from build123d import *
from OCP.BRepFilletAPI import BRepFilletAPI_MakeChamfer

# Parameters (mm, degrees)
BOSS_EXTRUDE1_DEPTH     = 23.2
BOSS_EXTRUDE2_START     = 23.2
BOSS_EXTRUDE2_DEPTH     = 75
CUT_EXTRUDE1_DEPTH      = 108.706127959
CUT_EXTRUDE1_DEPTH_BACK = 108.706127959
SKETCH2_W               = 2
SKETCH2_H               = 5
CUT_EXTRUDE2_DEPTH      = 108.706127959
CUT_EXTRUDE2_DEPTH_BACK = 108.706127959
CUT_EXTRUDE3_DEPTH      = 108.706127959
CUT_EXTRUDE3_DEPTH_BACK = 108.706127959
BOSS_EXTRUDE3_DEPTH     = 3.2
SKETCH5_W               = 84.2
SKETCH5_H               = 3.2
BOSS_EXTRUDE4_DEPTH     = 120
BOSS_EXTRUDE5_DEPTH     = 120
CUT_EXTRUDE4_DEPTH      = 136.132897549
CUT_EXTRUDE4_DEPTH_BACK = 136.132897549
CHAMFER1_SIZE           = 3.6
CHAMFER1_SIZE2          = 1.2
CHAMFER2_SIZE           = 1.2
FILLET1_R               = 0.8


with BuildPart() as part:
    # Sketch1 → Boss-Extrude1 (new body)
    with BuildSketch(Plane(origin=(0, 0, 0), x_dir=(1, 0, 0), z_dir=(0, 1, 0))):
        Polygon((-22.25475327, 13.6), (22.25475327, 13.6), (42.1, 10.359959718), (42.1, -10.359959718), (22.25475327, -13.6), (-22.25475327, -13.6), (-42.1, -10.359959718), (-42.1, 10.359959718), align=None)
    extrude(amount=BOSS_EXTRUDE1_DEPTH)

    # Sketch1<3> → Boss-Extrude2 (add)
    with BuildSketch(Plane(origin=(0, 0, 0), x_dir=(1, 0, 0), z_dir=(0, 1, 0)).offset(BOSS_EXTRUDE2_START)):
        Polygon((40.5, -9), (28.25, -11), (28.25, -8.9), (11, -8.9), (11, -12), (-11, -12), (-11, -8.9), (-28.25, -8.9), (-28.25, -11), (-40.5, -9), (-40.5, 9), (-28.25, 11), (-28.25, 8.9), (-11, 8.9), (-11, 12), (11, 12), (11, 8.9), (28.25, 8.9), (28.25, 11), (40.5, 9), align=None)
        Polygon((-38.9, -7.640040282), (-29.85, -9.117591303), (-29.85, -7.3), (-9.4, -7.3), (-9.4, -10.4), (9.4, -10.4), (9.4, -7.3), (29.85, -7.3), (29.85, -9.117591303), (38.9, -7.640040282), (38.9, 7.640040282), (29.85, 9.117591303), (29.85, 7.3), (9.4, 7.3), (9.4, 10.4), (-9.4, 10.4), (-9.4, 7.3), (-29.85, 7.3), (-29.85, 9.117591303), (-38.9, 7.640040282), align=None, mode=Mode.SUBTRACT)
    extrude(amount=BOSS_EXTRUDE2_DEPTH)

    # Sketch2 → Cut-Extrude1 (cut, two sides: drawn at the far end of the back side and taken through both)
    with BuildSketch(Plane.XY.offset(-CUT_EXTRUDE1_DEPTH_BACK)):
        with Locations((-39.5, 44.7)):
            Rectangle(SKETCH2_W, SKETCH2_H)
        with Locations((39.5, 44.7)):
            Rectangle(SKETCH2_W, SKETCH2_H)
    extrude(amount=CUT_EXTRUDE1_DEPTH + CUT_EXTRUDE1_DEPTH_BACK, mode=Mode.SUBTRACT)

    # Sketch3 → Cut-Extrude2 (cut, two sides: drawn at the far end of the back side and taken through both)
    with BuildSketch(Plane.XY.offset(-CUT_EXTRUDE2_DEPTH_BACK)):
        Polygon((-28.25, 93.2), (-19.625, 23.2), (19.625, 23.2), (28.25, 93.2), (28.25, 98.2), (-28.25, 98.2), align=None)
    extrude(amount=CUT_EXTRUDE2_DEPTH + CUT_EXTRUDE2_DEPTH_BACK, mode=Mode.SUBTRACT)

    # Sketch1<4> → Cut-Extrude3 (cut, two sides: drawn at the far end of the back side and taken through both)
    with BuildSketch(Plane(origin=(0, 0, 0), x_dir=(1, 0, 0), z_dir=(0, 1, 0)).offset(-CUT_EXTRUDE3_DEPTH_BACK)):
        Polygon((-31.45, -5.7), (-7.8, -5.7), (-7.8, -8.8), (7.8, -8.8), (7.8, -5.7), (31.45, -5.7), (31.45, -7.235182606), (37.3, -6.280080565), (37.3, 6.280080565), (31.45, 7.235182606), (31.45, 5.7), (7.8, 5.7), (7.8, 8.8), (-7.8, 8.8), (-7.8, 5.7), (-31.45, 5.7), (-31.45, 7.235182606), (-37.3, 6.280080565), (-37.3, -6.280080565), (-31.45, -7.235182606), align=None)
    extrude(amount=CUT_EXTRUDE3_DEPTH + CUT_EXTRUDE3_DEPTH_BACK, mode=Mode.SUBTRACT)

    # Sketch4 → Boss-Extrude3 (add)
    with BuildSketch(Plane(origin=(0, 0, 0), x_dir=(1, 0, 0), z_dir=(0, 1, 0))):
        Polygon((42.1, 10.359959718), (22.25475327, 13.6), (-22.25475327, 13.6), (-42.1, 10.359959718), (-42.1, 42.5), (42.1, 42.5), align=None)
    extrude(amount=BOSS_EXTRUDE3_DEPTH)

    # Sketch5 → Boss-Extrude4 (add)
    with BuildSketch(Plane(origin=(0, 0, 0), x_dir=(1, 0, 0), z_dir=(0, 1, 0))):
        with Locations((0, 44.1)):
            Rectangle(SKETCH5_W, SKETCH5_H)
    extrude(amount=BOSS_EXTRUDE4_DEPTH)

    # Sketch6 → Boss-Extrude5 (add)
    with BuildSketch(Plane(origin=(0, 0, 0), x_dir=(1, 0, 0), z_dir=(0, 1, 0))):
        Polygon((-42.1, 42.5), (42.1, 42.5), (28.25, 40.9), (-28.25, 40.9), align=None)
    extrude(amount=BOSS_EXTRUDE5_DEPTH)

    # Sketch7 → Cut-Extrude4 (cut, two sides: drawn at the far end of the back side and taken through both)
    with BuildSketch(Plane(origin=(0, 0, 0), x_dir=(-1, 0, 0), z_dir=(0, 0, -1)).offset(-CUT_EXTRUDE4_DEPTH_BACK)):
        with BuildLine():
            Line((-12, 67.5), (-12, 52.5))
            ThreePointArc((-12, 52.5), (-15, 49.5), (-18, 52.5))
            Line((-18, 52.5), (-18, 67.5))
            ThreePointArc((-18, 67.5), (-15, 70.5), (-12, 67.5))
        make_face()
        with BuildLine():
            Line((12, 67.5), (12, 52.5))
            ThreePointArc((12, 52.5), (15, 49.5), (18, 52.5))
            Line((18, 52.5), (18, 67.5))
            ThreePointArc((18, 67.5), (15, 70.5), (12, 67.5))
        make_face()
    extrude(amount=CUT_EXTRUDE4_DEPTH + CUT_EXTRUDE4_DEPTH_BACK, mode=Mode.SUBTRACT)

    # Chamfer1: one chamfer whose edges measure the first distance from different faces: ONE call of the kernel's chamfer builder (chamfer() names one face for all edges)
    chamfer1_edges_1 = [part.edges().sort_by_distance(p)[0] for p in [
        (35.175, 120, -41.7),
    ]]
    chamfer1_side_1 = [part.faces().sort_by_distance(p)[0] for p in [
        (35.175, 61.6, -41.7),
    ]]
    chamfer1_edges_2 = [part.edges().sort_by_distance(p)[0] for p in [
        (0, 120, -40.9),
    ]]
    chamfer1_side_2 = [part.faces().sort_by_distance(p)[0] for p in [
        (0, 61.659484301, -40.9),
    ]]
    chamfer1_edges_3 = [part.edges().sort_by_distance(p)[0] for p in [
        (-35.175, 120, -41.7),
    ]]
    chamfer1_side_3 = [part.faces().sort_by_distance(p)[0] for p in [
        (-35.175, 61.6, -41.7),
    ]]
    chamfer1 = BRepFilletAPI_MakeChamfer(part.part.solid().wrapped)
    for e in chamfer1_edges_1:
        chamfer1.Add(CHAMFER1_SIZE, CHAMFER1_SIZE2, e.wrapped, chamfer1_side_1[0].wrapped)  # the first distance lies on this face
    for e in chamfer1_edges_2:
        chamfer1.Add(CHAMFER1_SIZE, CHAMFER1_SIZE2, e.wrapped, chamfer1_side_2[0].wrapped)  # the first distance lies on this face
    for e in chamfer1_edges_3:
        chamfer1.Add(CHAMFER1_SIZE, CHAMFER1_SIZE2, e.wrapped, chamfer1_side_3[0].wrapped)  # the first distance lies on this face
    add(Compound.cast(chamfer1.Shape()), mode=Mode.REPLACE)

    # Chamfer2
    chamfer2_edges = [part.edges().sort_by_distance(p)[0] for p in [
        (-42.1, 0, -17.670020141),
        (-7.8, 23.2, 7.25),
        (7.8, 23.2, 7.25),
        (7.8, 23.2, -7.25),
        (-7.8, 23.2, -7.25),
        (-7.8, 0, -7.25),
        (-7.8, 0, 7.25),
        (40.5, 98.2, 0),
        (28.25, 98.2, -9.15),
        (0, 0, -45.7),
        (-28.25, 98.2, 9.15),
        (28.25, 98.2, 9.15),
        (-28.25, 98.2, -9.15),
        (-40.5, 98.2, 0),
        (-32.177376635, 0, 11.979979859),
        (0, 0, 13.6),
        (32.177376635, 0, 11.979979859),
        (42.1, 0, -17.670020141),
    ]]
    chamfer(chamfer2_edges, length=CHAMFER2_SIZE)

    # Fillet1
    fillet1_edges = [part.edges().sort_by_distance(p)[0] for p in [
        (-42.1, 12.2, 10.359959718),
        (42.1, 12.2, 10.359959718),
        (42.1, 13.2, -10.359959718),
        (-42.1, 13.2, -10.359959718),
        (-42.1, 60.6, -45.7),
        (42.1, 60.6, -45.7),
    ]]
    fillet(fillet1_edges, radius=FILLET1_R)


solid = part.part
Design review of the part built by this model. Coordinates are the model's own, in mm. A direction names the side the tool comes from. Coordinates: 2 decimals unless noted, no trailing zeros. Loops run counter-clockwise (first coordinate to the right, second up) from the corner with the lowest first, then second, coordinate; pieces in that order, holes last. Notation, with made-up numbers: (88, 59) -> (112, 59) arc R19 cw to (112, 68) -> close; hole circle Ø9 at (57.5, 65). An arc over 180 degrees is marked (long way). Use a Markdown table: item, result. Add a question column.
Item 1: The part is to be moulded in two halves that separate along X. For faces 1 (the flat face through (1, 3.2, -26)), 2 (the flat face through (-28.25, 60, -10)), 3 (the flat face through (-31.708, 12.046, 12.057)), say which applies: +X half, -X half, draft (parallel to the pull), parting line (faces both ways), or undercut.
Item 2: Wall thickness on L1, parallel to Z at x = 3, y = 7; L2, parallel to Z at x = -24.5, y = 47; L3, parallel to X at y = 19, z = -8: over which ranges is each line inside the solid? List them lowest first. Write a range as from..to.
Item 3: Clearance check with flat-ended pins moving along their axes: P1, Ø10, axis at x = -1, z = -4.5, coming from the -Y side; P2, Ø12, axis at x = 23, y = 59, coming from the +Z side; P3, Ø0.8, axis at y = 45, z = 8, coming from the +X side; P4, Ø0.9, axis at y = 54.5, z = 8, coming from the -X side. State where each tip first meets the part, or that it passes through.
Item 4: Machinability: for faces 4 (the flat face through (31.708, 13.06, -12.057)), 5 (the flat face through (40.5, 33, 0)), 6 (the flat face through (20, 11, -5.7)), which of the approach directions +Z, -Z, +X, -X, +Y, -Y give a long, thin tool a straight path to every point of the face, cutting with its end or side? Answer none if there is none.
Item 5: We need section A-A, the plane z = 0.5. Write out the cut boundary in (x, y).
Item 6: We need section D-D, the plane y = 82. Count the separate pieces of the cut face and the enclosed holes in it, and give its area (3 significant figures).
Item 7: We need section C-C, the plane x = -2.5. Write out the cut boundary in (y, z), and give its area (3 significant figures).
Item 8: We need section B-B, the plane x = 15. Write out the cut boundary in (y, z).
Numbers:
| question | item | result |
|---|---|---|
| 1 | face 1 | draft |
| 1 | face 2 | undercut |
| 1 | face 3 | -X half |
| 2 | L1 | z = -45.7..-40.9, -13.6..-8.8, 8.8..13.6 |
| 2 | L2 | z = -45.7..-40.9, -8.9..-7.3, 7.3..8.9 |
| 2 | L3 | x = -42.1..-7.8, 7.8..42.1 |
| 3 | P1 | stops at y = 0 |
| 3 | P2 | stops at z = 11 |
| 3 | P3 | stops at x = 38.5 |
| 3 | P4 | stops at x = -40.5 |
| 4 | face 4 | +X, +Y |
| 4 | face 5 | +Z, +X, +Y |
| 4 | face 6 | +Y, -Y |
| 5 | outline | (-42.1, 1.2) -> (-40.9, 0) -> (-37.3, 0) -> (-37.3, 23.2) -> (-38.9, 23.2) -> (-38.9, 42.2) -> (-40.5, 42.2) -> (-40.5, 23.2) -> (-42.1, 23.2) -> close; (-40.5, 47.2) -> (-38.9, 47.2) -> (-38.9, 98.2) -> (-39.3, 98.2) -> (-40.5, 97) -> close; (37.3, 0) -> (40.9, 0) -> (42.1, 1.2) -> (42.1, 23.2) -> (40.5, 23.2) -> (40.5, 42.2) -> (38.9, 42.2) -> (38.9, 23.2) -> (37.3, 23.2) -> close; (38.9, 47.2) -> (40.5, 47.2) -> (40.5, 97) -> (39.3, 98.2) -> (38.9, 98.2) -> close |
| 6 | separate pieces | 3 |
| 6 | enclosed holes | 0 |
| 6 | area | 531 mm^2 |
| 7 | outline | (0, -44.5) -> (1.2, -45.7) -> (120, -45.7) -> (120, -42.1) -> (116.4, -40.9) -> (3.2, -40.9) -> (3.2, -13.6) -> (23.2, -13.6) -> (23.2, -8.8) -> (0, -8.8) -> close; (0, 8.8) -> (23.2, 8.8) -> (23.2, 13.6) -> (1.2, 13.6) -> (0, 12.4) -> close |
| 7 | area | 882 mm^2 |
| 8 | outline | (0, -44.5) -> (1.2, -45.7) -> (49.5, -45.7) -> (49.5, -40.9) -> (3.2, -40.9) -> (3.2, -13.6) -> (23.2, -13.6) -> (23.2, -5.7) -> (0, -5.7) -> close; (0, 5.7) -> (23.2, 5.7) -> (23.2, 13.6) -> (1.2, 13.6) -> (0, 12.4) -> close; (70.5, -45.7) -> (120, -45.7) -> (120, -42.1) -> (116.4, -40.9) -> (70.5, -40.9) -> close |
